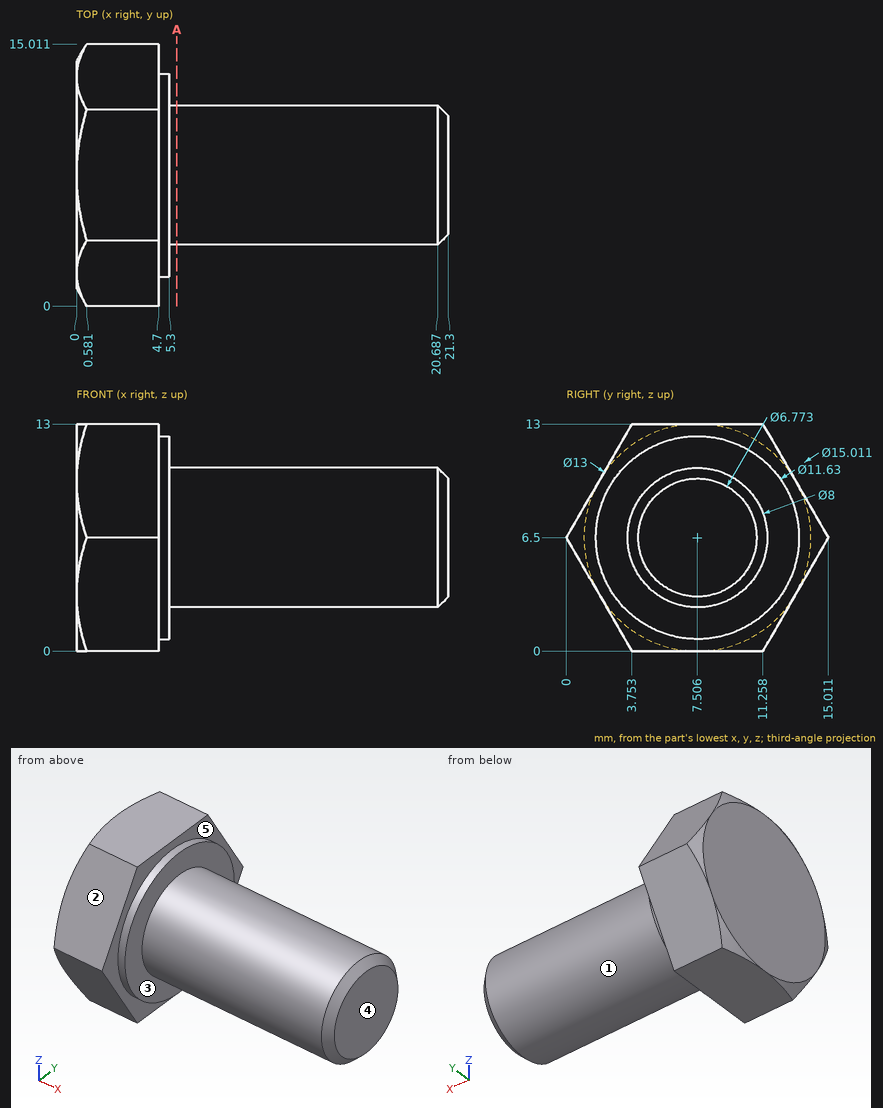
Source: three-view drawing plus pictorial views. Frame: mm from the lowest corner of the part. A direction names the side the tool comes from. Round coordinates to 2 decimals unless told otherwise and drop trailing zeros. Order: outer loops, then holes, each group sorted by start corner. A loop starts at its lowest first (then second) coordinate and runs counter-clockwise, first axis right, second up. Notation, with made-up numbers: (-24, 89.25) -> (0, 89.25) arc R33 ccw to (0, 119.25) -> close; hole circle Ø1 at (7, 70.5). An arc over 180 degrees is marked (long way). Use one line per item in the form item = value. Start each with the question number.
1. Pin query (flat end, axial travel): pin 1 Ø1.5 at (x, z) = (13, 8) entering from +Y (1 decimal); pin 2 Ø3 at (x, z) = (16.5, 6.5) entering from -Y; pin 3 Ø1 at (x, y) = (5.5, 9.5) entering from -Z; pin 4 Ø6 at (y, z) = (13.5, 11) entering from -X. Return the tip coordinate at first contact, or that it passes through.
2. Reachability of the marked faces 4 and 5 from +Z, -Z, +X, -X, +Y, -Y: full face, straight path, thin tool, end or side. Return the list, or none.
3. Cut plane A-A (x = 5.75). Return the cut outline in (y, z) (1 decimal).
4. Draft query along Z for the marked faces 1, 2 and 3. Return one class per face: pulls with the +Z half, pulls with the -Z half, needs draft (parallel to the pull), parting line crosses it, or undercut.
5. Line query: probe 1 along Z at (x, y) = (16.25, 7.5); probe 2 along X at (y, z) = (9.5, 11.75); probe 3 along Z at (x, y) = (12, 4.5). Output: solid intervals per line, ascending.
Solution:
q1.pin_1 = 11.4
q1.pin_2 = 3.51
q1.pin_3 = 0.89
q1.pin_4 = 0
q2.face_4 = +Z, -Z, +X, +Y, -Y
q2.face_5 = +X
q3.outline = circle Ø8 at (7.5, 6.5)
q4.face_1 = parting line crosses it
q4.face_2 = pulls with the +Z half
q4.face_3 = needs draft
q5.probe_1 = 2.5 to 10.5
q5.probe_2 = 0 to 5.3
q5.probe_3 = 3.86 to 9.14
